Geometry: final body of the model. Coordinates: model frame, mm. A direction names the side the tool comes from. Give positions to 0.01 mm unless a question says otherwise; leave off trailing zeros. Write each loop counter-clockwise with the first axis right and the second up, starting at its lowest first coordinate (ties: lowest second). Pieces come first, ordered by that corner, then holes.
from build123d import *

# Parameters (mm, degrees)
SKETCH1_R           = 20
SKETCH1_R_2         = 0.95
BOSS_EXTRUDE1_DEPTH = 2.5


with BuildPart() as part:
    # Sketch1 → Boss-Extrude1 (new body)
    with BuildSketch(Plane(origin=(0, 0, 0), x_dir=(1, 0, 0), z_dir=(0, 1, 0))):
        with Locations(Location((0, 0, 0), (0, 0, 270))):
            Circle(SKETCH1_R)
        with Locations(Location((0, 0, 0), (0, 0, 270))):
            Circle(SKETCH1_R_2, mode=Mode.SUBTRACT)
        with BuildLine():
            Line((-2.5, 3.75), (2.5, 3.75))
            Line((2.5, 3.75), (2.5, 18.75))
            ThreePointArc((2.5, 18.75), (0, 18.915932438), (-2.5, 18.75))
            Line((-2.5, 18.75), (-2.5, 3.75))
        make_face(mode=Mode.SUBTRACT)
        with BuildLine():
            Line((2.5, -3.75), (2.5, -18.75))
            ThreePointArc((2.5, -18.75), (0, -18.915932438), (-2.5, -18.75))
            Line((-2.5, -18.75), (-2.5, -3.75))
            Line((-2.5, -3.75), (2.5, -3.75))
        make_face(mode=Mode.SUBTRACT)
    extrude(amount=BOSS_EXTRUDE1_DEPTH)


solid = part.part
Q1. Access query for faces 4 (the flat face through (-2.5, 1, 11)), 5 (the flat face through (-4, 0, 0)). Directions: +Z, -Z, +X, -X, +Y, -Y. A direction counts if a zero-diameter tool reaches every point of the face in a straight line with its end or side. Return the directions, or none.
Filled sheet:
face 4: +Y, -Y
face 5: +Z, -Z, +X, -X, -Y
Q2. Pin query (flat end, axial travel): P1, Ø0.8, axis at y = 1.5, z = -11.5, coming from the +X side; P2, Ø2, axis at x = 0, z = 0, coming from the -Y side; P3, Ø0.8, axis at y = 1, z = 10.5, coming from the +X side; P4, Ø1.2, axis at x = -1, y = 1.5, coming from the -Z side. Return the tip coordinate at first contact, or that it passes through.
Filled sheet:
P1: stops at x = 16.64
P2: stops at y = 0
P3: stops at x = 17.26
P4: stops at z = -20
Q3. Section D-D on z = -11. Output: boundary loops of the cut face in (x, y), plus the area to 3 significant figures.
Filled sheet:
outline: (-16.7, 0) - (-2.5, 0) - (-2.5, 2.5) - (-16.7, 2.5) - close; (2.5, 0) - (16.7, 0) - (16.7, 2.5) - (2.5, 2.5) - close
area: 71.0 mm2
Q4. Ray query, line 1 along X through (y, z) = (1.45, 0); line 2 along X through (y, z) = (1.25, 4.5); line 3 along Z through (x, y) = (-16, 0.4). Return the intervals inside material, ascending.
Filled sheet:
line 1: x = -20 to -0.95, 0.95 to 20
line 2: x = -19.49 to -2.5, 2.5 to 19.49
line 3: z = -12 to 12
Q5. Pull-direction query (X, two-part tool) for faces 1 (the flat face through (0, 1, -3.75)), 2 (the flat face through (-4, 2.5, 0)), 3 (the cylindrical face through (-19.524, 1.232, -4.336)); classes: released by +X, released by -X, zero draft, split by the parting line, or undercut.
Filled sheet:
face 1: undercut
face 2: zero draft
face 3: split by the parting line
Q6. Section A-A on z = 0. Output: boundary loops of the cut face in (x, y), plus the area to 4 significant figures.
Filled sheet:
outline: (-20, 0) - (-0.95, 0) - (-0.95, 2.5) - (-20, 2.5) - close; (0.95, 0) - (20, 0) - (20, 2.5) - (0.95, 2.5) - close
area: 95.25 mm2
Q7. Section C-C on x = 0. Output: boundary loops of the cut face in (y, z).
Filled sheet:
outline: (0, -20) - (2.5, -20) - (2.5, -18.92) - (0, -18.92) - close; (0, -3.75) - (2.5, -3.75) - (2.5, -0.95) - (0, -0.95) - close; (0, 0.95) - (2.5, 0.95) - (2.5, 3.75) - (0, 3.75) - close; (0, 18.92) - (2.5, 18.92) - (2.5, 20) - (0, 20) - close
Q8. Section B-B on y = 0.9. Output: boundary loops of the cut face in (x, z), plus the area to 3 significant figures.
Filled sheet:
outline: circle Ø40 at (0, 0); hole (-2.5, -18.75) arc R18.92 ccw to (2.5, -18.75) - (2.5, -3.75) - (-2.5, -3.75) - close; hole (-2.5, 3.75) - (2.5, 3.75) - (2.5, 18.75) arc R18.92 ccw to (-2.5, 18.75) - close; hole circle Ø1.9 at (0, 0)
area: 1,100 mm2
